Solid Edge part; units mm, degrees
sketch "Sketch1" plane through (0, 0, 0) normal (0, -1, 0) x (1, 0, 0)
  line L0 (10, 10) -> (-10, 10)
  line L1 (-10, 10) -> (-10, -10)
  line L2 (-10, -10) -> (10, -10)
  line L3 (10, -10) -> (10, 10)
  circle A0 centre (-2.5, 0) radius 1
  circle A1 centre (0, 5) radius 1.5
  circle A2 centre (-5, -5) radius 1
  circle A3 centre (5, -5) radius 1
  circle A4 centre (2.5, 0) radius 1
extrude "Protrusion1" add sketch "Sketch1" against normal blind 2
sketch "Sketch2" plane through (0, 0, 0) normal (0, -1, 0) x (1, 0, 0)
  line L0 (7.5, 7.5) -> (-7.5, 7.5)
  line L1 (-7.5, 7.5) -> (-7.5, -7.5)
  line L2 (-7.5, -7.5) -> (7.5, -7.5)
  line L3 (7.5, -7.5) -> (7.5, 7.5)
  circle A0 centre (0, 5) radius 1.5
  circle A1 centre (-2.5, 0) radius 1
  circle A2 centre (2.5, 0) radius 1
  circle A3 centre (5, -5) radius 1
  circle A4 centre (-5, -5) radius 1
extrude "ExtrudedProtrusion_2" add sketch "Sketch2" along normal blind 0.25
sketch "Sketch3" plane through (0, -0.25, 0) normal (0, -1, 0) x (0, 0, 1)
  circle A0 centre (-5, 5) radius 1.1
  circle A1 centre (0, 2.5) radius 1.1
  circle A2 centre (0, -2.5) radius 1.1
  circle A3 centre (-5, -5.0202) radius 1.1
  circle A4 centre (5, 0) radius 1.6
extrude "ExtrudedCutout_1" cut sketch "Sketch3" against normal blind 1
sketch "Sketch4" plane through (0, -0.25, 0) normal (0, -1, 0) x (0, 0, 1)
  circle A0 centre (-9, 0) radius 0.6
  circle A1 centre (9, 0) radius 0.6
extrude "ExtrudedCutout_3" cut sketch "Sketch4" against normal blind 1
Can you work these out from the model? Positions are in its coordinate system, mm. A direction names the side the tool comes from. Give positions to 0.01 mm unless a question says otherwise; leave off trailing zeros. Loops run counter-clockwise (first coordinate to the right, second up) from the corner with the lowest first, then second, coordinate; pieces in that order, holes last. Notation, with made-up numbers: (48.25, -19) -> (80.25, -19) arc R18 ccw to (80.25, -4) -> close; hole circle Ø8 at (2, -28). An arc over 180 degrees is marked (long way). Write item = value, one per line.
1) Will this pin go through, and if not, where does the flat tip stop? pin 1 (1.3 mm diameter, centred on x = 0, z = -9, fed in from -Y).
Check result:
pin_1 = 0
2) Thinking about a two-plate mould opening in X: for faces 1 (the cylindrical face through (1.5, 1.4, 0)), 2 (the flat face through (0, 1, 10)), 3 (the flat face through (-10, 1, 0)), which applies, released by +X, released by -X, zero draft, split by the parting line, or undercut?
Check result:
face_1 = undercut
face_2 = zero draft
face_3 = released by -X
3) Suppose I cut it at D-D on z = 5. Write out the boundary of the cut face in (x, y).
Check result:
outline = (-10, 0) -> (-7.5, 0) -> (-7.5, -0.25) -> (-1.6, -0.25) -> (-1.6, 0.75) -> (-1.5, 0.75) -> (-1.5, 2) -> (-10, 2) -> close; (1.5, 0.75) -> (1.6, 0.75) -> (1.6, -0.25) -> (7.5, -0.25) -> (7.5, 0) -> (10, 0) -> (10, 2) -> (1.5, 2) -> close
4) For faces 4 (the cylindrical face through (0, 0.4, -9.6)), 5 (the flat face through (0, 2, 0)), which set-ups out of +Z, -Z, +X, -X, +Y, -Y let a thin tool reach every point of the face, with its end or its side?
Check result:
face_4 = -Y
face_5 = +Z, -Z, +X, -X, +Y
5) I need wall thicknesses on L1, parallel to X at y = 0.1, z = -5; L2, parallel to Z at x = 0, y = 0.3; L3, parallel to Z at x = -2.5, y = 1.4. Which ranges of each line are inside material? Lowest first, please. Write a range as from..to.
Check result:
L1 = -10..-6.1, -3.9..3.92, 6.12..10
L2 = -10..-9.6, -8.4..3.4, 6.6..8.4, 9.6..10
L3 = -10..-1, 1..10
6) Suppose I cut it at A-A on z = -5. Write out the boundary of the cut face in (x, y), then the cut area to 4 significant figures.
Check result:
outline = (-10, 0) -> (-7.5, 0) -> (-7.5, -0.25) -> (-6.1, -0.25) -> (-6.1, 0.75) -> (-6, 0.75) -> (-6, 2) -> (-10, 2) -> close; (-4, 0.75) -> (-3.9, 0.75) -> (-3.9, -0.25) -> (3.92, -0.25) -> (3.92, 0.75) -> (4, 0.75) -> (4, 2) -> (-4, 2) -> close; (6, 0.75) -> (6.12, 0.75) -> (6.12, -0.25) -> (7.5, -0.25) -> (7.5, 0) -> (10, 0) -> (10, 2) -> (6, 2) -> close
area = 34.35 mm2
7) Suppose I cut it at C-C on x = -2.5. Write out the boundary of the cut face in (y, z).
Check result:
outline = (-0.25, -7.5) -> (0, -7.5) -> (0, -10) -> (2, -10) -> (2, -1) -> (0.75, -1) -> (0.75, -1.1) -> (-0.25, -1.1) -> close; (-0.25, 1.1) -> (0.75, 1.1) -> (0.75, 1) -> (2, 1) -> (2, 10) -> (0, 10) -> (0, 7.5) -> (-0.25, 7.5) -> close
8) Suppose I cut it at B-B on y = 1.3. Write out the boundary of the cut face in (x, z).
Check result:
outline = (-10, -10) -> (10, -10) -> (10, 10) -> (-10, 10) -> close; hole circle Ø2 at (-5, -5); hole circle Ø2 at (-2.5, 0); hole circle Ø3 at (0, 5); hole circle Ø2 at (2.5, 0); hole circle Ø2 at (5, -5)
